```python
from build123d import *

# Parameters (mm, degrees)
BOSS_EXTRUDE1_DEPTH      = 8.5
BOSS_EXTRUDE1_DEPTH_BACK = 8.5
SKETCH1_W                = 72
SKETCH1_H                = 28.5
SKETCH2_W                = 31.201469113
SKETCH2_H                = 12
CUT_EXTRUDE1_DEPTH       = 69
SKETCH3_W                = 10
SKETCH3_H                = 17
BOSS_EXTRUDE2_DEPTH      = 3
CUT_EXTRUDE2_DEPTH       = 10
FILLET1_R                = 1
BOSS_EXTRUDE3_DEPTH      = 2
SKETCH8_W                = 12.8
SKETCH8_H                = 12.8
SKETCH8_R                = 3.26
SKETCH8_R_2              = 2.4
CUT_EXTRUDE3_DEPTH       = 2
SKETCH11_W               = 26
SKETCH11_H               = 12
BOSS_EXTRUDE7_DEPTH      = 3.1
SKETCH14_R               = 1
CUT_EXTRUDE4_DEPTH       = 62.43948242
CUT_EXTRUDE6_DEPTH       = 62.43948242
CUT_EXTRUDE7_DEPTH       = 62.43948242
BOSS_EXTRUDE8_DEPTH      = 14
SKETCH19_R               = 1
CUT_EXTRUDE8_DEPTH       = 5
SKETCH20_W               = 17.87603411
SKETCH20_H               = 5.867107887
CUT_EXTRUDE9_DEPTH       = 62.686708455
FILLET4_R                = 1
CUT_EXTRUDE10_DEPTH      = 10
BOSS_EXTRUDE9_START      = 1.4
BOSS_EXTRUDE9_DEPTH      = 1.4
FILLET5_R                = 0.2


with BuildPart() as part:
    # Sketch1 → Boss-Extrude1 (new, two sides: drawn at the far end of the back side and taken through both)
    with BuildSketch(Plane(origin=(0, 0, 0), x_dir=(1, 0, 0), z_dir=(0, 1, 0)).offset(-BOSS_EXTRUDE1_DEPTH_BACK)):
        with Locations((0, 14.25)):
            Rectangle(SKETCH1_W, SKETCH1_H)
    extrude(amount=BOSS_EXTRUDE1_DEPTH + BOSS_EXTRUDE1_DEPTH_BACK)

    # Sketch2 → Cut-Extrude1 (cut)
    with BuildSketch(Plane.ZY.offset(36)):
        with Locations((-10.899265443, 0)):
            Rectangle(SKETCH2_W, SKETCH2_H)
    extrude(amount=-CUT_EXTRUDE1_DEPTH, mode=Mode.SUBTRACT)

    # Sketch3 → Boss-Extrude2 (add)
    with BuildSketch(Plane.XY):
        with Locations((31, 0)):
            Rectangle(SKETCH3_W, SKETCH3_H)
    extrude(amount=-BOSS_EXTRUDE2_DEPTH)

    # Sketch6 → Cut-Extrude2 (cut)
    with BuildSketch(Plane(origin=(0, 0, -28.5), x_dir=(-1, 0, 0), z_dir=(0, 0, -1))):
        Polygon((-11, 8.5), (-11, 5.5), (-8, 5.5), (-8, 8), (8, 8), (8, 5.5), (11, 5.5), (11, 8.5), align=None)
        Polygon((-11, -5.5), (-11, -8.5), (11, -8.5), (11, -5.5), (8, -5.5), (8, -8), (-8, -8), (-8, -5.5), align=None)
    extrude(amount=-CUT_EXTRUDE2_DEPTH, mode=Mode.SUBTRACT)

    # Fillet1
    # the kernel refuses this fillet: 1 mm, written as the material it adds along each edge
    with BuildSketch(Plane(origin=(-8, -8, -18.5), x_dir=(0, 0, -1), z_dir=(1, 0, 0)), Plane(origin=(8, 8, -18.5), x_dir=(0, 0, -1), z_dir=(-1, 0, 0))) as fillet1_piece_1:
        with BuildLine():
            CenterArc((0.866025404, -1), FILLET1_R, 90, 60)
            Line((0, -0.5), (-0.017320508, -0.49))
            ThreePointArc((-0.017320508, -0.49), (-0.02, -0.25), (-0.02, 0))
            Line((-0.02, 0), (0, 0.02))
            Line((0, 0.02), (0.866025404, 0.02))
            Line((0.866025404, 0.02), (0.866025404, 0))
        make_face()
    extrude(amount=16)

    # Sketch7 → Boss-Extrude3 (add)
    with BuildSketch(Plane.XY.offset(-26.5)):
        Polygon((33, -6), (33, 6), (11, 6), (11, 5.5), (8, 5.5), (8, 6), (-8, 6), (-8, 5.5), (-11, 5.5), (-11, 6), (-13, 6), (-13, -6), (-11, -6), (-11, -5.5), (-8, -5.5), (-8, -6), (8, -6), (8, -5.5), (11, -5.5), (11, -6), align=None)
    extrude(amount=BOSS_EXTRUDE3_DEPTH)

    # Sketch8 → Cut-Extrude3 (cut)
    # profile 1 of 2: a face of its own
    with BuildSketch(Plane(origin=(0, 0, -28.5), x_dir=(-1, 0, 0), z_dir=(0, 0, -1))):
        Rectangle(SKETCH8_W, SKETCH8_H)
        Circle(SKETCH8_R, mode=Mode.SUBTRACT)
    # profile 2 of 2: a face of its own
    with BuildSketch(Plane(origin=(0, 0, -28.5), x_dir=(-1, 0, 0), z_dir=(0, 0, -1))):
        Circle(SKETCH8_R_2)
    extrude(amount=-CUT_EXTRUDE3_DEPTH, mode=Mode.SUBTRACT)

    # Sketch11 → Boss-Extrude7 (add)
    with BuildSketch(Plane.XY.offset(3.1)):
        with Locations((39, 0)):
            Rectangle(SKETCH11_W, SKETCH11_H)
    extrude(amount=-BOSS_EXTRUDE7_DEPTH)

    # Sketch14 → Cut-Extrude4 (cut, through all)
    with BuildSketch(Plane.XY.offset(3.1)):
        with Locations((41, 0)):
            Circle(SKETCH14_R)
    extrude(amount=-CUT_EXTRUDE4_DEPTH, mode=Mode.SUBTRACT)

    # Sketch15 → Cut-Extrude6 (cut, through all)
    with BuildSketch(Plane.XY.offset(3.1)):
        with BuildLine():
            Line((52, 6), (36, 6))
            Line((36, 6), (49.658536622, 2.92682926))
            ThreePointArc((49.658536622, 2.92682926), (51.34260644, 1.874085128), (52, 0))
            Line((52, 0), (52, 6))
        make_face()
    extrude(amount=-CUT_EXTRUDE6_DEPTH, mode=Mode.SUBTRACT)

    # Sketch17 → Cut-Extrude7 (cut, through all)
    with BuildSketch(Plane.XY.offset(3.1)):
        with BuildLine():
            Line((36, -6), (52, -6))
            Line((52, -6), (52, 0))
            ThreePointArc((52, 0), (51.342606414, -1.874085161), (49.658536541, -2.926829278))
            Line((49.658536541, -2.926829278), (36, -6))
        make_face()
    extrude(amount=-CUT_EXTRUDE7_DEPTH, mode=Mode.SUBTRACT)

    # Sketch18 → Boss-Extrude8 (add)
    with BuildSketch(Plane.XY.offset(-24.5)):
        Polygon((-11, 6), (-13, 6), (-13, -6), (-11, -6), (-11, -5.5), (-8, -5.5), (-8, 5.5), (-11, 5.5), align=None)
    extrude(amount=BOSS_EXTRUDE8_DEPTH)

    # Sketch19 → Cut-Extrude8 (cut)
    with BuildSketch(Plane.XY.offset(-10.5)):
        with Locations((-10.25, 0)):
            Circle(SKETCH19_R)
    extrude(amount=-CUT_EXTRUDE8_DEPTH, mode=Mode.SUBTRACT)

    # Sketch20 → Cut-Extrude9 (cut, through all)
    with BuildSketch(Plane.XZ.offset(8.5)):
        with Locations((44.938017055, -2.033553943)):
            Rectangle(SKETCH20_W, SKETCH20_H)
    extrude(amount=-CUT_EXTRUDE9_DEPTH, mode=Mode.SUBTRACT)

    # Fillet4
    # the kernel refuses this fillet: 1 mm, written as the material it adds along each edge
    with BuildSketch(Plane(origin=(36, -8.5, 0.9), x_dir=(1, 0, 0), z_dir=(0, 1, 0))) as fillet4_piece_1_section:
        with BuildLine():
            CenterArc((FILLET4_R, FILLET4_R), FILLET4_R, 180, 90)
            Line((0, FILLET4_R), (0, 0))
            Line((0, 0), (FILLET4_R, 0))
        make_face()
    fillet4_piece_1 = extrude(amount=14.5, mode=Mode.PRIVATE)
    fillet4_piece_1 = split(fillet4_piece_1, bisect_by=Plane(origin=(35.990889593, -7.251037957, 0), z_dir=(0, 0, -1)), keep=Keep.TOP, mode=Mode.PRIVATE)
    fillet4_piece_1 = split(fillet4_piece_1, bisect_by=Plane(origin=(35.723408497, -6.062233088, -0.048071683), z_dir=(0.21951219512195128, -0.9756097560975611, 0)), keep=Keep.TOP, mode=Mode.PRIVATE)
    fillet4_piece_1 = split(fillet4_piece_1, bisect_by=Plane(origin=(35.990889593, -6, -0.048071683), z_dir=(0, -1, 0)), keep=Keep.TOP, mode=Mode.PRIVATE)
    add(fillet4_piece_1)
    with BuildSketch(Plane(origin=(36, -6, 0.9), x_dir=(1, 0, 0), z_dir=(0, 1, 0))) as fillet4_piece_2_section:
        with BuildLine():
            CenterArc((FILLET4_R, FILLET4_R), FILLET4_R, 180, 90)
            Line((0, FILLET4_R), (0, 0))
            Line((0, 0), (FILLET4_R, 0))
        make_face()
    fillet4_piece_2 = extrude(amount=12, mode=Mode.PRIVATE)
    fillet4_piece_2 = split(fillet4_piece_2, bisect_by=Plane(origin=(36.226665296, 0, 0), z_dir=(0, 0, 1)), keep=Keep.TOP, mode=Mode.PRIVATE)
    fillet4_piece_2 = split(fillet4_piece_2, bisect_by=Plane(origin=(37.500692727, 5.662344136, 0.678804193), z_dir=(-0.2195121951219508, -0.9756097560975612, 0)), keep=Keep.TOP, mode=Mode.PRIVATE)
    fillet4_piece_2 = split(fillet4_piece_2, bisect_by=Plane(origin=(37.500692727, -5.662344136, 0.678804193), z_dir=(-0.21951219512195128, 0.9756097560975611, 0)), keep=Keep.TOP, mode=Mode.PRIVATE)
    add(fillet4_piece_2)
    with BuildSketch(Plane(origin=(36, -6, 0.9), x_dir=(1, 0, 0), z_dir=(0, 1, 0))) as fillet4_piece_3_section:
        with BuildLine():
            CenterArc((FILLET4_R, FILLET4_R), FILLET4_R, 180, 90)
            Line((0, FILLET4_R), (0, 0))
            Line((0, 0), (FILLET4_R, 0))
        make_face()
    fillet4_piece_3 = extrude(amount=12, mode=Mode.PRIVATE)
    fillet4_piece_3 = split(fillet4_piece_3, bisect_by=Plane(origin=(35.990886035, 0, 0), z_dir=(0, 0, -1)), keep=Keep.TOP, mode=Mode.PRIVATE)
    add(fillet4_piece_3)
    with BuildSketch(Plane(origin=(36, -6, 0.9), x_dir=(1, 0, 0), z_dir=(0, 1, 0))) as fillet4_piece_4_section:
        with BuildLine():
            CenterArc((FILLET4_R, FILLET4_R), FILLET4_R, 180, 90)
            Line((0, FILLET4_R), (0, 0))
            Line((0, 0), (FILLET4_R, 0))
        make_face()
    fillet4_piece_4 = extrude(amount=14.5, mode=Mode.PRIVATE)
    fillet4_piece_4 = split(fillet4_piece_4, bisect_by=Plane(origin=(35.990889593, 7.251037957, 0), z_dir=(0, 0, -1)), keep=Keep.TOP, mode=Mode.PRIVATE)
    fillet4_piece_4 = split(fillet4_piece_4, bisect_by=Plane(origin=(35.990889593, 6, -0.048071683), z_dir=(0, 1, 0)), keep=Keep.TOP, mode=Mode.PRIVATE)
    fillet4_piece_4 = split(fillet4_piece_4, bisect_by=Plane(origin=(35.723408497, 6.062233088, -0.048071683), z_dir=(0.2195121951219508, 0.9756097560975612, 0)), keep=Keep.TOP, mode=Mode.PRIVATE)
    add(fillet4_piece_4)

    # Sketch21 → Cut-Extrude10 (cut)
    with BuildSketch(Plane.XY.offset(3.1)):
        with BuildLine():
            ThreePointArc((48.87804878, 0), (48.028247344, -2.422597855), (45.851279032, -3.783462218))
            Line((45.851279032, -3.783462218), (49.658536585, -2.926829268))
            ThreePointArc((49.658536585, -2.926829268), (52, 0), (49.658536585, 2.926829268))
            Line((49.658536585, 2.926829268), (45.851279024, 3.78346222))
            ThreePointArc((45.851279024, 3.78346222), (48.028247342, 2.422597858), (48.87804878, 0))
        make_face()
    extrude(amount=-CUT_EXTRUDE10_DEPTH, mode=Mode.SUBTRACT)

    # Sketch23 → Boss-Extrude9 (add)
    with BuildSketch(Plane.XY.offset(3.1).offset(BOSS_EXTRUDE9_START)):
        with BuildLine():
            ThreePointArc((40.896590916, -2.397771165), (38.6, -8e-09), (40.896590899, 2.397771165))
            Line((40.896590899, 2.397771165), (47.78858717, 2.695003514))
            ThreePointArc((47.78858717, 2.695003514), (46.899563641, 3.380964406), (45.851279001, 3.783462225))
            Line((45.851279001, 3.783462225), (36, 6))
            Line((36, 6), (26, 6))
            Line((26, 6), (26, -6))
            Line((26, -6), (36, -6))
            Line((36, -6), (45.851279001, -3.783462225))
            ThreePointArc((45.851279001, -3.783462225), (46.899563641, -3.380964406), (47.78858717, -2.695003514))
            Line((47.78858717, -2.695003514), (40.896590916, -2.397771165))
        make_face()
    extrude(amount=-BOSS_EXTRUDE9_DEPTH)

    # Fillet5
    fillet5_edges = [part.edges().sort_by_distance(p)[0] for p in [
        (47.78858717, 2.695003514, 3.8),
        (47.78858717, -2.695003514, 3.8),
    ]]
    fillet(fillet5_edges, radius=FILLET5_R)


solid = part.part
```
Verification items for the finished model (mm, model axes). A direction names the side the tool comes from. Round coordinates to 2 decimals unless told otherwise and drop trailing zeros. Write each loop counter-clockwise with the first axis right and the second up, starting at its lowest first coordinate (ties: lowest second). Pieces come first, ordered by that corner, then holes. Notation, with made-up numbers: (50, 89.25) - (106, 89.25) arc R17 cw to (106, 98.25) - close; hole circle Ø8 at (-36.75, 50.5). An arc over 180 degrees is marked (long way). Answer as a JSON object with one key per item and string values. Group by question number.
Q1. Go/stop test with flat-tipped pins: pin 1 Ø2 at (x, y) = (1, -7) entering from +Z; pin 2 Ø3.5 at (y, z) = (-2, -21) entering from +X; pin 3 Ø2.5 at (x, z) = (10, -26.5) entering from -Y; pin 4 Ø8 at (y, z) = (-0.5, -3) entering from -X. Record where each tip stops, or that it passes through.
Q2. Mould release check, pull along X, two halves, no side actions. Record for faces 5 (the flat face through (11, -7, -24)), 6 (the flat face through (43, 0, 0.9)), 7 (the cylindrical face through (38.6, -0.05, 3.81)): released by +X, released by -X, zero draft, split by the parting line, or undercut.
Q3. Section check B-B, the plane z = -22. Enter the section's corners in (x, y), plus the area to 3 significant figures.
Q4. Thickness scan on line 1 (Y direction, x = 14, z = -9.5); line 2 (X direction, y = 2.75, z = -13.5); line 3 (Z direction, x = 30, y = 2.5). Record the ranges inside material, lowest first.
Q5. Tool access check on faces 1 (the flat face through (11, 7, -24)), 2 (the flat face through (33, 0, -14)), 3 (the flat face through (-10, -5.5, -20)), 4 (the cylindrical face through (-1.75, 2.75, -27.51)). Record the directions out of +Z, -Z, +X, -X, +Y, -Y that give a thin tool (end or side, any length) a straight path to the whole face; none if there is none.
Q6. Section check D-D, the plane x = -29. Enter the section's corners in (y, z).
Q7. Section check C-C, the plane z = -14. Enter the section's corners in (x, y).
Q8. Section check A-A, the plane x = -10.25. Enter the section's corners in (y, z).
Found:
{
 "1": {"pin 1": "stops at z = 0", "pin 2": "stops at x = 36", "pin 3": "stops at y = -8.5", "pin 4": "stops at x = 26"},
 "2": {"face 5": "undercut", "face 6": "zero draft", "face 7": "released by +X"},
 "3": {"outline": "(-36, -8.5) - (-11, -8.5) - (-11, -5.5) - (-8, -5.5) - (-8, 5.5) - (-11, 5.5) - (-11, 8.5) - (-36, 8.5) - (-36, 6) - (-13, 6) - (-13, -6) - (-36, -6) - close; (-8, -8) - (8, -8) - (8, -6) - (-8, -6) - close; (-8, 6) - (8, 6) - (8, 8) - (-8, 8) - close; (11, -8.5) - (36, -8.5) - (36, 8.5) - (11, 8.5) - (11, 6) - (33, 6) - (33, -6) - (11, -6) - close", "area": "407 mm^2"},
 "4": {"line 1": "y = -8.5 to -6, 6 to 8.5", "line 2": "x = -13 to -8, 33 to 36", "line 3": "z = -28.5 to -24.5, -3 to 4.5"},
 "5": {"face 1": "-Z, +Y", "face 2": "none", "face 3": "+Z, -Z", "face 4": "-Z"},
 "6": {"outline": "(-8.5, -28.5) - (8.5, -28.5) - (8.5, 0) - (6, 0) - (6, -26.5) - (-6, -26.5) - (-6, 0) - (-8.5, 0) - close"},
 "7": {"outline": "(-36, -8.5) - (36, -8.5) - (36, 8.5) - (-36, 8.5) - (-36, 6) - (-13, 6) - (-13, -6) - (-36, -6) - close; hole circle Ø2 at (-10.25, 0); hole (-11, -6) - (33, -6) - (33, 6) - (-11, 6) - (-11, 5.5) - (-8, 5.5) - (-8, -5.5) - (-11, -5.5) - close"},
 "8": {"outline": "(-8.5, -18.5) - (-6, -18.5) - (-6, 0) - (-8.5, 0) - close; (-5.5, -28.5) - (5.5, -28.5) - (5.5, -10.5) - (1, -10.5) - (1, -15.5) - (-1, -15.5) - (-1, -10.5) - (-5.5, -10.5) - close; (6, -18.5) - (8.5, -18.5) - (8.5, 0) - (6, 0) - close"}
}
